Build history of the part. All positions in model axes, mm. Face numbers are marked on the shaded views. A direction names the side the tool comes from. Round coordinates to 2 decimals unless told otherwise and drop trailing zeros. Loops run counter-clockwise (first coordinate to the right, second up) from the corner with the lowest first, then second, coordinate; pieces in that order, holes last. Notation, with made-up numbers: (77.25, 57.5) - (102.25, 57.5) arc R27 ccw to (102.25, 74.5) - close; hole circle Ø5 at (-25.75, 59). An arc over 180 degrees is marked (long way). Use one line per item in the form item = value. Start each with the question number.
Q1. 3-axis set-ups, long thin cutter, end or side, ignore diameter. For the marked faces 1, 2, 3 and 4: which of +Z, -Z, +X, -X, +Y, -Y reach the whole face in a straight line?
Q2. Pin check, flat tips, straight feed: pin 1 (1 mm diameter, centred on x = -23.5, z = 19, fed in from -Y); pin 2 (12 mm diameter, centred on x = 43, z = 30.5, fed in from -Y); pin 3 (4 mm diameter, centred on x = -2, y = 41, fed in from +Z). Stop position of each tip, or through.
Q3. Saw through at B-B (x = 2.5). Give the cut face in (y, z).
Q4. Saw through at A-A (z = 8). Give the cut face in (x, y).
Q5. Saw through at C-C (y = 3). Give the cut face in (x, z).
Q6. Saw through at D-D (z = 35). Give the cut face in (x, y) (1 decimal), then the cut area to 3 significant figures.
Q7. Drill centre lines: line 1 (X direction, y = 30, z = 32); line 2 (X direction, y = -21, z = 24.5); line 3 (X direction, y = -14, z = 15.5). Where is each one in solid material? Low to high.
Q8. Mould opens along X. For the marked faces 5, 6 and 7 say: released by +X, released by -X, zero draft, split by the parting line, or undercut.
```python
from build123d import *

# Parameters (mm, degrees)
F0_R     = 7.5
F1_DEPTH = 2
F2_DEPTH = 40
F4_DEPTH = 10


with BuildPart() as f1:
    # F0 (on Top) → F1 (new body)
    with BuildSketch(Plane.XY):
        with BuildLine():
            ThreePointArc((60.856366, -24.384369), (36.710284, -7.376819), (10.3731, 5.988912))
            ThreePointArc((10.3731, 5.988912), (11.966629, 35.480448), (9.3107, 64.895344))
            ThreePointArc((9.3107, 64.895344), (0, 67.2), (-9.3107, 64.895344))
            ThreePointArc((-9.3107, 64.895344), (-11.966629, 35.480448), (-10.3731, 5.988912))
            ThreePointArc((-10.3731, 5.988912), (-36.710284, -7.376819), (-60.856366, -24.384369))
            ThreePointArc((-60.856366, -24.384369), (-58.196907, -33.6), (-51.545666, -40.510974))
            ThreePointArc((-51.545666, -40.510974), (-24.743655, -28.103629), (0, -11.977824))
            ThreePointArc((0, -11.977824), (24.743655, -28.103629), (51.545666, -40.510974))
            ThreePointArc((51.545666, -40.510974), (58.196907, -33.6), (60.856366, -24.384369))
        make_face()
        with BuildLine():
            ThreePointArc((-7.5, 63.559028), (0, 65.2), (7.5, 63.559028))
            ThreePointArc((7.5, 63.559028), (9.985947, 34.169463), (8.191847, 4.729565))
            ThreePointArc((8.191847, 4.729565), (34.584597, -8.436648), (58.793733, -25.284323))
            ThreePointArc((58.793733, -25.284323), (56.464856, -32.6), (51.293733, -38.274704))
            ThreePointArc((51.293733, -38.274704), (24.59865, -25.732816), (0, -9.45913))
            ThreePointArc((0, -9.45913), (-24.59865, -25.732816), (-51.293733, -38.274704))
            ThreePointArc((-51.293733, -38.274704), (-56.464856, -32.6), (-58.793733, -25.284323))
            ThreePointArc((-58.793733, -25.284323), (-34.584597, -8.436648), (-8.191847, 4.729565))
            ThreePointArc((-8.191847, 4.729565), (-9.985947, 34.169463), (-7.5, 63.559028))
        make_face(mode=Mode.SUBTRACT)
        with BuildLine():
            ThreePointArc((8.191847, 4.729565), (9.985947, 34.169463), (7.5, 63.559028))
            ThreePointArc((7.5, 63.559028), (0, 65.2), (-7.5, 63.559028))
            ThreePointArc((-7.5, 63.559028), (-9.985947, 34.169463), (-8.191847, 4.729565))
            ThreePointArc((-8.191847, 4.729565), (-34.584597, -8.436648), (-58.793733, -25.284323))
            ThreePointArc((-58.793733, -25.284323), (-56.464856, -32.6), (-51.293733, -38.274704))
            ThreePointArc((-51.293733, -38.274704), (-24.59865, -25.732816), (0, -9.45913))
            ThreePointArc((0, -9.45913), (24.59865, -25.732816), (51.293733, -38.274704))
            ThreePointArc((51.293733, -38.274704), (56.464856, -32.6), (58.793733, -25.284323))
            ThreePointArc((58.793733, -25.284323), (34.584597, -8.436648), (8.191847, 4.729565))
        make_face()
        Circle(F0_R, mode=Mode.SUBTRACT)
        Circle(F0_R)
    extrude(amount=-F1_DEPTH)

    # F0 (on Top) → F2 (join)
    with BuildSketch(Plane.XY):
        with BuildLine():
            ThreePointArc((60.856366, -24.384369), (36.710284, -7.376819), (10.3731, 5.988912))
            ThreePointArc((10.3731, 5.988912), (11.966629, 35.480448), (9.3107, 64.895344))
            ThreePointArc((9.3107, 64.895344), (0, 67.2), (-9.3107, 64.895344))
            ThreePointArc((-9.3107, 64.895344), (-11.966629, 35.480448), (-10.3731, 5.988912))
            ThreePointArc((-10.3731, 5.988912), (-36.710284, -7.376819), (-60.856366, -24.384369))
            ThreePointArc((-60.856366, -24.384369), (-58.196907, -33.6), (-51.545666, -40.510974))
            ThreePointArc((-51.545666, -40.510974), (-24.743655, -28.103629), (0, -11.977824))
            ThreePointArc((0, -11.977824), (24.743655, -28.103629), (51.545666, -40.510974))
            ThreePointArc((51.545666, -40.510974), (58.196907, -33.6), (60.856366, -24.384369))
        make_face()
        with BuildLine():
            ThreePointArc((-7.5, 63.559028), (0, 65.2), (7.5, 63.559028))
            ThreePointArc((7.5, 63.559028), (9.985947, 34.169463), (8.191847, 4.729565))
            ThreePointArc((8.191847, 4.729565), (34.584597, -8.436648), (58.793733, -25.284323))
            ThreePointArc((58.793733, -25.284323), (56.464856, -32.6), (51.293733, -38.274704))
            ThreePointArc((51.293733, -38.274704), (24.59865, -25.732816), (0, -9.45913))
            ThreePointArc((0, -9.45913), (-24.59865, -25.732816), (-51.293733, -38.274704))
            ThreePointArc((-51.293733, -38.274704), (-56.464856, -32.6), (-58.793733, -25.284323))
            ThreePointArc((-58.793733, -25.284323), (-34.584597, -8.436648), (-8.191847, 4.729565))
            ThreePointArc((-8.191847, 4.729565), (-9.985947, 34.169463), (-7.5, 63.559028))
        make_face(mode=Mode.SUBTRACT)
    extrude(amount=F2_DEPTH)

    # F3 (on face) → F4 (cut)
    with BuildSketch(Plane.XY.offset(40)):
        with BuildLine():
            ThreePointArc((-51.545666, -40.510974), (-24.743655, -28.103629), (0, -11.977824))
            ThreePointArc((0, -11.977824), (24.743655, -28.103629), (51.545666, -40.510974))
            ThreePointArc((51.545666, -40.510974), (58.196907, -33.6), (60.856366, -24.384369))
            ThreePointArc((60.856366, -24.384369), (36.710284, -7.376819), (10.3731, 5.988912))
            ThreePointArc((10.3731, 5.988912), (11.966629, 35.480448), (9.3107, 64.895344))
            ThreePointArc((9.3107, 64.895344), (0, 67.2), (-9.3107, 64.895344))
            ThreePointArc((-9.3107, 64.895344), (-11.966629, 35.480448), (-10.3731, 5.988912))
            ThreePointArc((-10.3731, 5.988912), (-36.710284, -7.376819), (-60.856366, -24.384369))
            ThreePointArc((-60.856366, -24.384369), (-58.196907, -33.6), (-51.545666, -40.510974))
        make_face()
        with BuildLine():
            ThreePointArc((51.451933, -39.619813), (24.689038, -27.158291), (0, -10.972078))
            ThreePointArc((0, -10.972078), (-24.689038, -27.158291), (-51.451933, -39.619813))
            ThreePointArc((-51.451933, -39.619813), (-57.504087, -33.2), (-60.037731, -24.748774))
            ThreePointArc((-60.037731, -24.748774), (-35.864289, -7.802188), (-9.502098, 5.486039))
            ThreePointArc((-9.502098, 5.486039), (-11.175251, 34.960479), (-8.585798, 64.368588))
            ThreePointArc((-8.585798, 64.368588), (0, 66.4), (8.585798, 64.368588))
            ThreePointArc((8.585798, 64.368588), (11.175251, 34.960479), (9.502098, 5.486039))
            ThreePointArc((9.502098, 5.486039), (35.864289, -7.802188), (60.037731, -24.748774))
            ThreePointArc((60.037731, -24.748774), (57.504087, -33.2), (51.451933, -39.619813))
        make_face(mode=Mode.SUBTRACT)
    extrude(amount=-F4_DEPTH, mode=Mode.SUBTRACT)


solid = f1.part
```
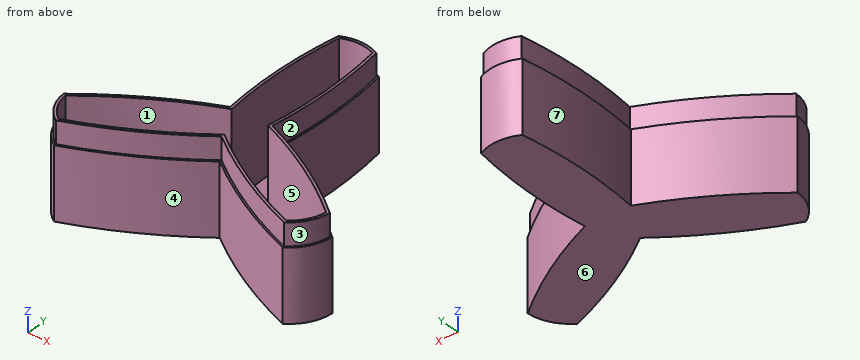
Report:
q1.face_1 = +Z
q1.face_2 = +Z, +X
q1.face_3 = +Z, +X, -Y
q1.face_4 = +Z, -Z, -Y
q2.pin_1 = -27.69
q2.pin_2 = -39.52
q2.pin_3 = 0
q3.outline = (-13.85, -2) - (67.04, -2) - (67.04, 30) - (66.24, 30) - (66.24, 40) - (65.03, 40) - (65.03, 0) - (-11.36, 0) - (-11.36, 40) - (-12.85, 40) - (-12.85, 30) - (-13.85, 30) - close
q4.outline = (-60.86, -24.38) arc R19.96 ccw to (-51.55, -40.51) arc R205.24 ccw to (0, -11.98) arc R205.24 ccw to (51.55, -40.51) arc R19.96 ccw to (60.86, -24.38) arc R205.24 ccw to (10.37, 5.99) arc R205.24 ccw to (9.31, 64.9) arc R19.96 ccw to (-9.31, 64.9) arc R205.24 ccw to (-10.37, 5.99) arc R205.24 ccw to start; hole (-58.79, -25.28) arc R17.96 ccw to (-51.29, -38.27) arc R203.24 ccw to (0, -9.46) arc R203.24 ccw to (51.29, -38.27) arc R17.96 ccw to (58.79, -25.28) arc R203.24 ccw to (8.19, 4.73) arc R203.24 ccw to (7.5, 63.56) arc R17.96 ccw to (-7.5, 63.56) arc R203.24 ccw to (-8.19, 4.73) arc R203.24 ccw to start
q5.outline = (-17.15, -2) - (17.15, -2) - (17.15, 30) - (15.22, 30) - (15.22, 40) - (12.27, 40) - (12.27, 0) - (-12.27, 0) - (-12.27, 40) - (-15.22, 40) - (-15.22, 30) - (-17.15, 30) - close
q6.outline = (-60, -24.7) arc R19.2 ccw to (-51.5, -39.6) arc R204.4 ccw to (0, -11) arc R204.4 ccw to (51.5, -39.6) arc R19.2 ccw to (60, -24.7) arc R204.4 ccw to (9.5, 5.5) arc R204.4 ccw to (8.6, 64.4) arc R19.2 ccw to (-8.6, 64.4) arc R204.4 ccw to (-9.5, 5.5) arc R204.4 ccw to start; hole (-58.8, -25.3) arc R18 ccw to (-51.3, -38.3) arc R203.2 ccw to (0, -9.5) arc R203.2 ccw to (51.3, -38.3) arc R18 ccw to (58.8, -25.3) arc R203.2 ccw to (8.2, 4.7) arc R203.2 ccw to (7.5, 63.6) arc R18 ccw to (-7.5, 63.6) arc R203.2 ccw to (-8.2, 4.7) arc R203.2 ccw to start
q6.area = 485 mm²
q7.line_1 = -11.19 to -9.99, 9.99 to 11.19
q7.line_2 = -56.61 to -53.31, -16.61 to -12.87, 12.87 to 16.61, 53.31 to 56.61
q7.line_3 = -47.01 to -43.44, -6.12 to -2.71, 2.71 to 6.12, 43.44 to 47.01
q8.face_5 = undercut
q8.face_6 = zero draft
q8.face_7 = released by -X
